Autodesk Inventor part; units mm, degrees
ref_plane "Plano de trabajo1" through (2.5, 0, 0) normal (1, 0, 0) x (0, 1, 0)
ref_plane "XZ Plane" through (0, 0, 0) normal (0, 1, 0) x (-1, 0, 0)
ref_plane "XY Plane" through (0, 0, 0) normal (0, 0, 1) x (1, 0, 0)
sketch "Boceto1" plane through (0, 0, 0) normal (0, 1, 0) x (-1, 0, 0)
  arc A0 (-2.5, 0) -> (2.5, 0) centre (0, 0) ccw
  line L0 (-2.5, 0) -> (2.5, 0)
  dimension "d0" = 5
revolve "Revolución1" add sketch "Boceto1" angle 360 about axis through (2.5, 0, 0) along (-1, 0, 0)
ref_plane "Plano de trabajo1" through (2.5, 0, 0) normal (1, 0, 0) x (0, 1, 0)
sketch "Boceto2" plane through (2.5, 0, 0) normal (1, 0, 0) x (0, 1, 0)
  circle A0 centre (0, 0) radius 1.5
  circle A1 centre (0, 0) radius 1.9
  dimension "d3" = 3
  dimension "d4" = 3.8
extrude "Extrusión1" add sketch "Boceto2" along normal blind 1 and the other way blind 6
sketch "Boceto3" plane through (2.5, 0, 0) normal (1, 0, 0) x (0, 1, 0)
  circle A0 centre (0, 0) radius 1.5
extrude "Extrusión2" cut sketch "Boceto3" against normal blind 10000
fillet "Empalme1" radius 0.08 2 edges at (-3.5, -1.5, 0) (3.5, -1.5, 0)
properties part number "Bola_libertad_grande"
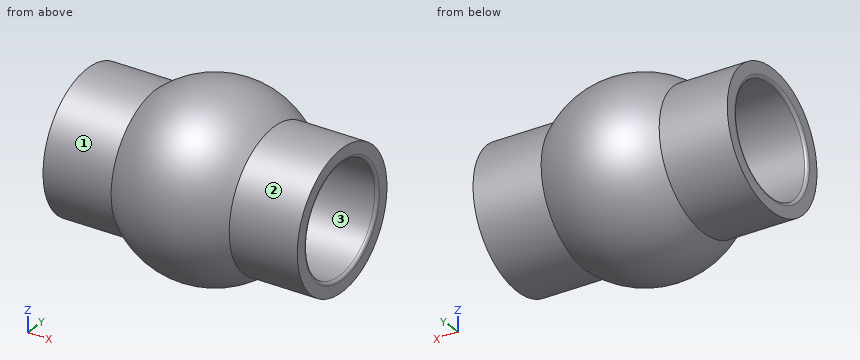
Verification items for the finished model (mm, model axes). Face numbers are marked on the shaded views. A direction names the side the tool comes from. Give positions to 0.01 mm unless a question says otherwise; leave off trailing zeros. Write each loop counter-clockwise with the first axis right and the second up, starting at its lowest first coordinate (ties: lowest second). Pieces come first, ordered by that corner, then holes. Notation, with made-up numbers: (6, -5.75) - (62, -5.75) arc R23 ccw to (62, 19.25) - close; hole circle Ø8 at (52, 89). An arc over 180 degrees is marked (long way). Answer as CSV lines item,"result". Start each with the question number.
1. Thickness scan on line 1 (Z direction, x = 2, y = 0); line 2 (Z direction, x = -1.25, y = 0); line 3 (Y direction, x = -1, z = 0.65). Record the ranges inside material, lowest first.
2. Sectioned sample at C-C (x = -2.25). Record the boundary of the cut face in (y, z).
3. Depth check by flat-ended pin: pin 1 (1.5 mm diameter, centred on x = -2.5, y = -0.5, fed in from +Z); pin 2 (3 mm diameter, centred on x = 1.5, z = -1.5, fed in from +Y); pin 3 (2 mm diameter, centred on x = -2.5, z = 0, fed in from -Y). Enter the tip coordinate at first touch or a pass-through.
4. Set-up check for the marked faces 1, 2 and 3: record each of +Z, -Z, +X, -X, +Y, -Y from which the full face is reachable in a straight line by a thin tool's end or side.
5. Sectioned sample at A-A (z = 0). Record the boundary of the cut face in (x, y), then the cut area to 3 significant figures.
Derived:
1,line 1,"-1.9 to -1.5, 1.5 to 1.9"
1,line 2,"-2.17 to -1.5, 1.5 to 2.17"
1,line 3,"-2.2 to -1.35, 1.35 to 2.2"
2,outline,"circle Ø3.8 at (0, 0); hole circle Ø3 at (0, 0)"
3,pin 1,"z = 1.9"
3,pin 2,"y = 2.42"
3,pin 3,"y = -2"
4,face 1,"-X"
4,face 2,"+X"
4,face 3,"+X, -X"
5,outline,"(-3.5, -1.9) - (-1.62, -1.9) arc R2.5 ccw to (1.62, -1.9) - (3.5, -1.9) - (3.5, -1.58) arc R0.08 ccw to (3.42, -1.5) - (-3.42, -1.5) arc R0.08 ccw to (-3.5, -1.58) - close; (-3.5, 1.58) arc R0.08 ccw to (-3.42, 1.5) - (3.42, 1.5) arc R0.08 ccw to (3.5, 1.58) - (3.5, 1.9) - (1.62, 1.9) arc R2.5 ccw to (-1.62, 1.9) - (-3.5, 1.9) - close"
5,area,"8.26 mm²"
